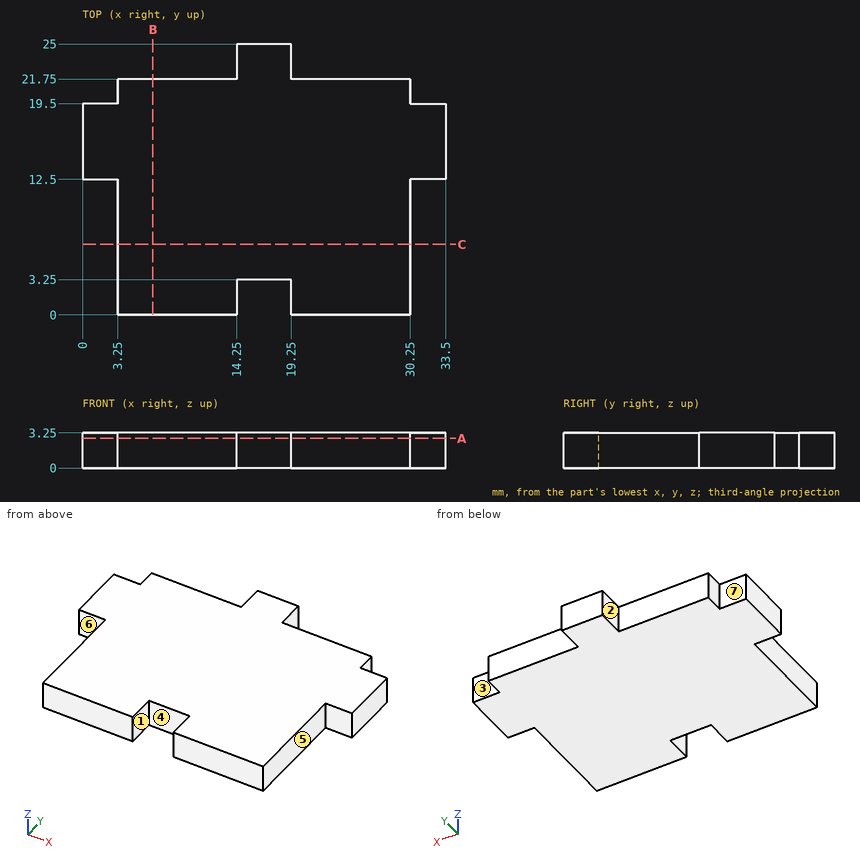
Check sheet for the drawn part. Datum: minimum x, y, z corner. Units: mm. A direction names the side the tool comes from. Round coordinates to 2 decimals unless told otherwise and drop trailing zeros. Loops run counter-clockwise (first coordinate to the right, second up) from the corner with the lowest first, then second, coordinate; pieces in that order, holes last. Notation, with made-up numbers: M -10,2 L 28,2 A17 ccw 28,8 Z; hole C -18,51.25 d11. An arc over 180 degrees is marked long. One line per question, with ' | ' between items. Start each with the question number.
Item 1: Section check A-A (z = 2.75). Record the boundary of the cut face in (x, y).
Item 2: Gauge pin test, flat ends, axial feed: pin 1 Ø1.6 at (y, z) = (2, 2) entering from +X; pin 2 Ø1.1 at (y, z) = (21, 2) entering from -X; pin 3 Ø1 at (x, z) = (31.5, 2.5) entering from -Y. Record the tip position at first contact, or that the pin passes through.
Item 3: Section check B-B (x = 6.5). Record the boundary of the cut face in (y, z).
Item 4: Release check for a two-part mould opening along X. For the marked faces 1, 2, 3 and 4 record: released by +X, released by -X, zero draft, split by the parting line, or undercut.
Item 5: Scan lines: probe 1 along X at (y, z) = (2, 1.5); probe 2 along Y at (x, z) = (22.5, 1.8); probe 3 along X at (y, z) = (9, 0.6). Record each from-to range of solid material in increasing order.
Item 6: Set-up check for the marked faces 5, 6 and 7: record each of +Z, -Z, +X, -X, +Y, -Y from which the full face is reachable in a straight line by a thin tool's end or side.
Item 7: Section check C-C (y = 6.5). Record the boundary of the cut face in (x, z), and give its area (4 significant figures).
Worked out:
1) outline: M 0,12.5 L 3.25,12.5 L 3.25,0 L 14.25,0 L 14.25,3.25 L 19.25,3.25 L 19.25,0 L 30.25,0 L 30.25,12.5 L 33.5,12.5 L 33.5,19.5 L 30.25,19.5 L 30.25,21.75 L 19.25,21.75 L 19.25,25 L 14.25,25 L 14.25,21.75 L 3.25,21.75 L 3.25,19.5 L 0,19.5 Z
2) pin 1: x = 30.25 | pin 2: x = 3.25 | pin 3: y = 12.5
3) outline: M 0,0 L 21.75,0 L 21.75,3.25 L 0,3.25 Z
4) face 1: undercut | face 2: released by -X | face 3: zero draft | face 4: undercut
5) probe 1: 3.25 to 14.25, 19.25 to 30.25 | probe 2: 0 to 21.75 | probe 3: 3.25 to 30.25
6) face 5: +Z, -Z, +X, -Y | face 6: +Z, -Z, -X, -Y | face 7: +Z, -Z, -X, +Y
7) outline: M 3.25,0 L 30.25,0 L 30.25,3.25 L 3.25,3.25 Z | area: 87.75 mm^2
